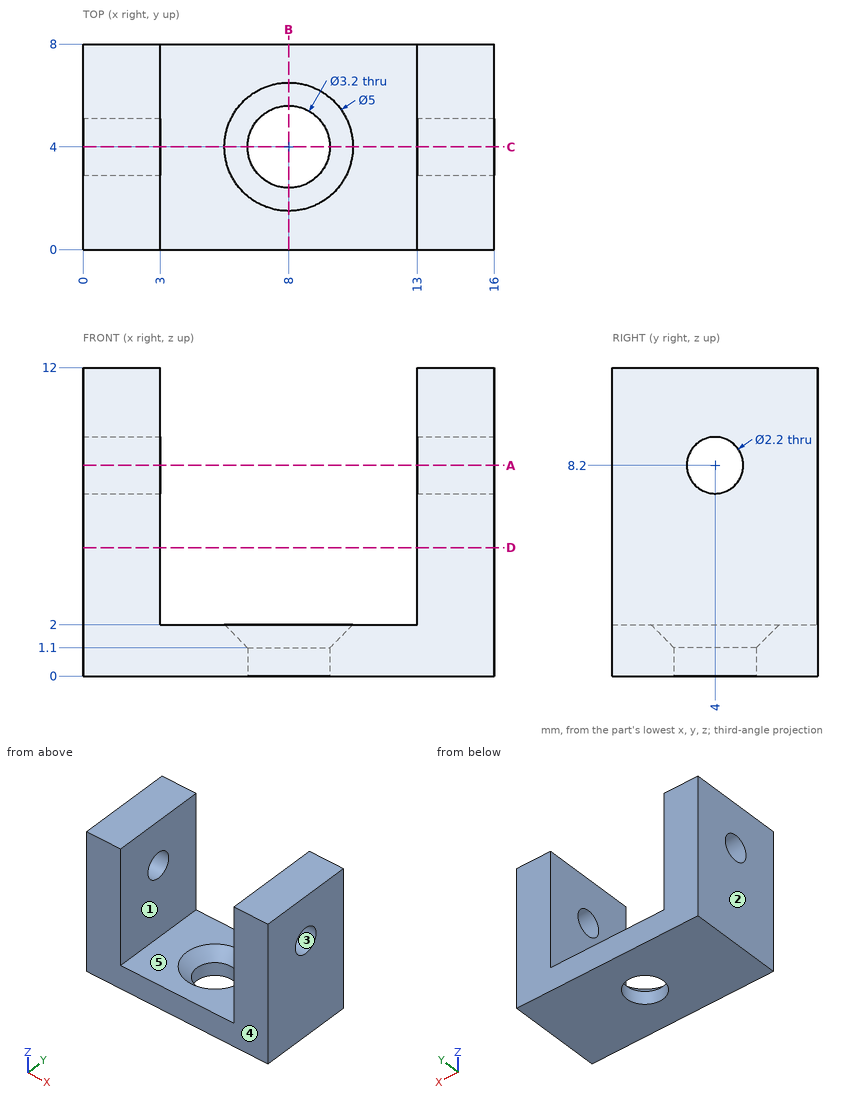
Geometry: see drawing. Coordinates: mm, zero at the bounding-box minimum. A direction names the side the tool comes from. Give positions to 0.01 mm unless a question says otherwise; leave off trailing zeros. Order: outer loops, then holes, each group sorted by start corner. A loop starts at its lowest first (then second) coordinate and runs counter-clockwise, first axis right, second up. Notation, with made-up numbers: (44.5, -3) - (100.5, -3) arc R28 ccw to (100.5, 36) - close; hole circle Ø5 at (-37.75, 34.5). An arc over 180 degrees is marked (long way). Use a Markdown table: item, result.
(1) Line query: line 1 (X direction, y = 4, z = 0.3); line 2 (X direction, y = 7.75, z = 6); line 3 (Z direction, x = 14.1, y = 4). Output: solid intervals per line, ascending. Write a range as from..to.
Computed values:
| item | result |
|---|---|
| line 1 | x = 0..6.4, 9.6..16 |
| line 2 | x = 0..3, 13..16 |
| line 3 | z = 0..7.1, 9.3..12 |
(2) Draft query along X for the marked faces 1, 2 and 3. Return one class per face: released by +X, released by -X, zero draft, split by the parting line, or undercut.
Computed values:
| item | result |
|---|---|
| face 1 | undercut |
| face 2 | released by -X |
| face 3 | zero draft |
(3) Section query D-D (z = 5). Output: boundary loops of the cut face in (x, y).
Computed values:
| item | result |
|---|---|
| outline | (0, 0) - (3, 0) - (3, 8) - (0, 8) - close; (13, 0) - (16, 0) - (16, 8) - (13, 8) - close |
(4) Access query for the marked faces 4 and 5. Directions: +Z, -Z, +X, -X, +Y, -Y. A direction counts if a zero-diameter tool reaches every point of the face in a straight line with its end or side. Return the directions, or none.
Computed values:
| item | result |
|---|---|
| face 4 | +Z, -Z, +X, -X, -Y |
| face 5 | +Z, +Y, -Y |
(5) Section query B-B (x = 8). Output: boundary loops of the cut face in (y, z), then the cut area to 3 significant figures.
Computed values:
| item | result |
|---|---|
| outline | (0, 0) - (2.4, 0) - (2.4, 1.1) - (1.5, 2) - (0, 2) - close; (5.6, 0) - (8, 0) - (8, 2) - (6.5, 2) - (5.6, 1.1) - close |
| area | 8.79 mm2 |
(6) Pin query (flat end, axial travel): pin 1 (1.3 mm diameter, centred on y = 4, z = 8.2, fed in from +X); pin 2 (1 mm diameter, centred on x = 4, y = 5.5, fed in from +Z); pin 3 (3.5 mm diameter, centred on x = 8, y = 4, fed in from +Z). Return the tip coordinate at first contact, or that it passes through.
Computed values:
| item | result |
|---|---|
| pin 1 | passes through |
| pin 2 | stops at z = 2 |
| pin 3 | stops at z = 1.25 |
(7) Section query A-A (z = 8.2). Output: boundary loops of the cut face in (x, y).
Computed values:
| item | result |
|---|---|
| outline | (0, 0) - (3, 0) - (3, 2.9) - (0, 2.9) - close; (0, 5.1) - (3, 5.1) - (3, 8) - (0, 8) - close; (13, 0) - (16, 0) - (16, 2.9) - (13, 2.9) - close; (13, 5.1) - (16, 5.1) - (16, 8) - (13, 8) - close |
(8) Section query C-C (y = 4). Output: boundary loops of the cut face in (x, z), then the cut area to 3 significant figures.
Computed values:
| item | result |
|---|---|
| outline | (0, 0) - (6.4, 0) - (6.4, 1.1) - (5.5, 2) - (3, 2) - (3, 7.1) - (0, 7.1) - close; (0, 9.3) - (3, 9.3) - (3, 12) - (0, 12) - close; (9.6, 0) - (16, 0) - (16, 7.1) - (13, 7.1) - (13, 2) - (10.5, 2) - (9.6, 1.1) - close; (13, 9.3) - (16, 9.3) - (16, 12) - (13, 12) - close |
| area | 71.6 mm2 |
